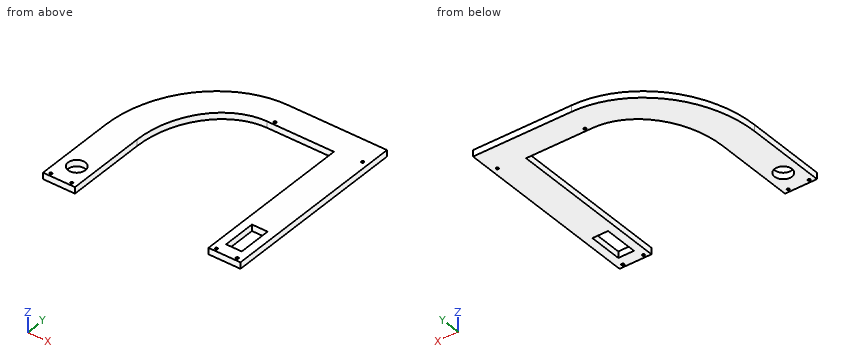
```python
from build123d import *

# Parameters (mm, degrees)
SKETCH2_W           = 246.38
SKETCH2_H           = 254
BOSS_EXTRUDE1_DEPTH = 7.9375
CUT_EXTRUDE2_REACH  = 9.938
SCREW_HOLES_REACH   = 9.938
SKETCH4_R           = 1.5875
CUT_EXTRUDE4_REACH  = 9.938
SKETCH5_R           = 10.795
CUT_EXTRUDE5_REACH  = 9.938
SKETCH6_W           = 19.558
SKETCH6_H           = 41.91


with BuildPart() as part:
    # Sketch2 → Boss-Extrude1 (new body)
    with BuildSketch(Plane.XY):
        with Locations((123.19, 127)):
            Rectangle(SKETCH2_W, SKETCH2_H)
    extrude(amount=BOSS_EXTRUDE1_DEPTH)

    # Sketch3 → Cut-Extrude2 (cut, up to next)
    with BuildSketch(Plane.XY.offset(7.9375), mode=Mode.PRIVATE) as cut_extrude2_sk1:
        with BuildLine():
            Line((0, 254), (0, 100.875137361))
            add(Edge.make_bspline(
                [(123.19, 237.422544345), (0, 237.422544345), (0, 100.875137361)],
                knots=[0, 0, 0, 1.570796327, 1.570796327, 1.570796327], degree=2, weights=[1, 0.707106781, 1]))
            Line((123.19, 237.422544345), (246.38, 237.422544345))
            Line((246.38, 237.422544345), (246.38, 254))
            Line((246.38, 254), (0, 254))
        make_face()
    cut_extrude2_tool1 = extrude(cut_extrude2_sk1.sketch, amount=-CUT_EXTRUDE2_REACH, mode=Mode.PRIVATE) & part.part
    add(cut_extrude2_tool1.solids().sort_by_distance((2.900868, 177.437569, 7.9375))[0], mode=Mode.SUBTRACT)
    # Sketch3 → Cut-Extrude2 (cut, up to next)
    with BuildSketch(Plane.XY.offset(7.9375), mode=Mode.PRIVATE) as cut_extrude2_sk2:
        with BuildLine():
            Line((39.878, 0), (39.878, 100.875137361))
            add(Edge.make_bspline(
                [(123.19, 203.2), (39.878, 203.2), (39.878, 100.875137361)],
                knots=[0, 0, 0, 1.570796327, 1.570796327, 1.570796327], degree=2, weights=[1, 0.707106781, 1]))
            Line((123.19, 203.2), (206.502, 203.2))
            Line((206.502, 203.2), (206.502, 160.284632983))
            Line((206.502, 160.284632983), (206.502, 0))
            Line((206.502, 0), (39.878, 0))
        make_face()
    cut_extrude2_tool2 = extrude(cut_extrude2_sk2.sketch, amount=-CUT_EXTRUDE2_REACH, mode=Mode.PRIVATE) & part.part
    add(cut_extrude2_tool2.solids().sort_by_distance((126.885795, 97.102181, 7.9375))[0], mode=Mode.SUBTRACT)

    # Sketch4 → screw holes (cut, up to next)
    with BuildSketch(Plane.XY.offset(7.9375), mode=Mode.PRIVATE) as screw_holes_sk1:
        with Locations((6.985, 3.81)):
            Circle(SKETCH4_R)
    screw_holes_tool1 = extrude(screw_holes_sk1.sketch, amount=-SCREW_HOLES_REACH, mode=Mode.PRIVATE) & part.part
    add(screw_holes_tool1.solids().sort_by_distance((6.985, 3.81, 7.9375))[0], mode=Mode.SUBTRACT)
    # Sketch4 → screw holes (cut, up to next)
    with BuildSketch(Plane.XY.offset(7.9375), mode=Mode.PRIVATE) as screw_holes_sk2:
        with Locations((32.893, 3.81)):
            Circle(SKETCH4_R)
    screw_holes_tool2 = extrude(screw_holes_sk2.sketch, amount=-SCREW_HOLES_REACH, mode=Mode.PRIVATE) & part.part
    add(screw_holes_tool2.solids().sort_by_distance((32.893, 3.81, 7.9375))[0], mode=Mode.SUBTRACT)
    # Sketch4 → screw holes (cut, up to next)
    with BuildSketch(Plane.XY.offset(7.9375), mode=Mode.PRIVATE) as screw_holes_sk3:
        with Locations((213.487, 3.81)):
            Circle(SKETCH4_R)
    screw_holes_tool3 = extrude(screw_holes_sk3.sketch, amount=-SCREW_HOLES_REACH, mode=Mode.PRIVATE) & part.part
    add(screw_holes_tool3.solids().sort_by_distance((213.487, 3.81, 7.9375))[0], mode=Mode.SUBTRACT)
    # Sketch4 → screw holes (cut, up to next)
    with BuildSketch(Plane.XY.offset(7.9375), mode=Mode.PRIVATE) as screw_holes_sk4:
        with Locations((239.395, 3.81)):
            Circle(SKETCH4_R)
    screw_holes_tool4 = extrude(screw_holes_sk4.sketch, amount=-SCREW_HOLES_REACH, mode=Mode.PRIVATE) & part.part
    add(screw_holes_tool4.solids().sort_by_distance((239.395, 3.81, 7.9375))[0], mode=Mode.SUBTRACT)
    # Sketch4 → screw holes (cut, up to next)
    with BuildSketch(Plane.XY.offset(7.9375), mode=Mode.PRIVATE) as screw_holes_sk5:
        with Locations((130.175, 207.01)):
            Circle(SKETCH4_R)
    screw_holes_tool5 = extrude(screw_holes_sk5.sketch, amount=-SCREW_HOLES_REACH, mode=Mode.PRIVATE) & part.part
    add(screw_holes_tool5.solids().sort_by_distance((130.175, 207.01, 7.9375))[0], mode=Mode.SUBTRACT)
    # Sketch4 → screw holes (cut, up to next)
    with BuildSketch(Plane.XY.offset(7.9375), mode=Mode.PRIVATE) as screw_holes_sk6:
        with Locations((239.395, 207.01)):
            Circle(SKETCH4_R)
    screw_holes_tool6 = extrude(screw_holes_sk6.sketch, amount=-SCREW_HOLES_REACH, mode=Mode.PRIVATE) & part.part
    add(screw_holes_tool6.solids().sort_by_distance((239.395, 207.01, 7.9375))[0], mode=Mode.SUBTRACT)

    # Sketch5 → Cut-Extrude4 (cut, up to next)
    with BuildSketch(Plane.XY.offset(7.9375), mode=Mode.PRIVATE) as cut_extrude4_sk1:
        with Locations((19.939, 28.702)):
            Circle(SKETCH5_R)
    cut_extrude4_tool1 = extrude(cut_extrude4_sk1.sketch, amount=-CUT_EXTRUDE4_REACH, mode=Mode.PRIVATE) & part.part
    add(cut_extrude4_tool1.solids().sort_by_distance((19.939, 28.702, 7.9375))[0], mode=Mode.SUBTRACT)

    # Sketch6 → Cut-Extrude5 (cut, up to next)
    with BuildSketch(Plane.XY.offset(7.9375), mode=Mode.PRIVATE) as cut_extrude5_sk1:
        with Locations((226.441, 36.195)):
            Rectangle(SKETCH6_W, SKETCH6_H)
    cut_extrude5_tool1 = extrude(cut_extrude5_sk1.sketch, amount=-CUT_EXTRUDE5_REACH, mode=Mode.PRIVATE) & part.part
    add(cut_extrude5_tool1.solids().sort_by_distance((226.441, 36.195, 7.9375))[0], mode=Mode.SUBTRACT)


solid = part.part
```
Design review of the part built by this model. Coordinates are the model's own, in mm. Coordinates: 2 decimals unless noted, no trailing zeros. Order: outer loops, then holes, each group sorted by start corner. A loop starts at its lowest first (then second) coordinate and runs counter-clockwise, first axis right, second up.
1) Take a section at A-A, the plane y = 77.5. Give the boundary of the cut face in (x, z), and give its area (3 significant figures).
2) Take a section at B-B, the plane z = 1.5. State how many separate pieces and enclosed holes the cut face has, and give its area (3 significant figures).
3) Wall thickness on line 1 along X through (y, z) = (16, 5.5); line 2 along X through (y, z) = (89, 0.75); line 3 along Y through (x, z) = (195.5, 7): over which ranges is each line inside the solid? List them lowest first.
4) Clearance check with flat-ended pins moving along their axes: pin 1 (4 mm diameter, centred on x = 164, z = 4.5, fed in from -Y); pin 2 (4 mm diameter, centred on x = 204, y = 189, fed in from -Z); pin 3 (1 mm diameter, centred on x = 60, z = 6, fed in from -Y). State where each tip first meets the part, or that it passes through.
Returned:
1. outline: (0, 0) - (39.88, 0) - (39.88, 7.94) - (0, 7.94) - close; (206.5, 0) - (246.38, 0) - (246.38, 7.94) - (206.5, 7.94) - close
1. area: 633 mm2
2. separate pieces: 1
2. enclosed holes: 8
2. area: 21,600 mm2
3. line 1: x = 0 to 39.88, 206.5 to 216.66, 236.22 to 246.38
3. line 2: x = 0 to 39.88, 206.5 to 246.38
3. line 3: y = 203.2 to 237.42
4. pin 1: stops at y = 203.2
4. pin 2: passes through
4. pin 3: stops at y = 166.84
